Check sheet for the modelled part. Datum: model origin and axes. Units: mm. Face numbers are marked on the shaded views. A direction names the side the tool comes from. Give positions to 0.01 mm unless a question says otherwise; leave off trailing zeros. Order: outer loops, then holes, each group sorted by start corner. A loop starts at its lowest first (then second) coordinate and runs counter-clockwise, first axis right, second up. Notation, with made-up numbers: (-15, -4.5) -> (12, -4.5) arc R35 ccw to (12, 34.5) -> close; hole circle Ø7 at (21.5, 38). An arc over 180 degrees is marked (long way). Answer in a Markdown table with one row per item. Add a question column.
(1) Cross-section at B-B (x = 8.5). Record the cut outline in (y, z).
(2) Release check for a two-part mould opening along X. For the marked faces 1, 2, 3 and 4 record: released by +X, released by -X, zero draft, split by the parting line, or undercut.
(3) Cross-section at D-D (x = 3.5). Record the cut outline in (y, z), then the cut area to 3 significant figures.
(4) Set-up check for the marked faces 5, 6, 7 and 8: record each of +Z, -Z, +X, -X, +Y, -Y from which the full face is reachable in a straight line by a thin tool's end or side.
(5) Cross-section at C-C (z = 5). Record the cut outline in (x, y), then the cut area to 3 significant figures.
(6) Go/stop test with flat-tipped pins: pin 1 (3.5 mm diameter, centred on x = 6, y = -0.5, fed in from +Z); pin 2 (1 mm diameter, centred on x = 8, y = 13.5, fed in from -Z); pin 3 (1 mm diameter, centred on x = 6.5, y = 13.5, fed in from +Z). Record where each tip stops, or that it passes through.
(7) Cross-section at A-A (y = 0). Record the cut outline in (x, z), then the cut area to 3 significant figures.
(8) Thickness scan on L1, parallel to Z at x = 8, y = 0.5; L2, parallel to Z at x = 8.5, y = -3; L3, parallel to Y at x = 8, z = 5. Record the ranges inside material, lowest first. Write a range as [from, to].
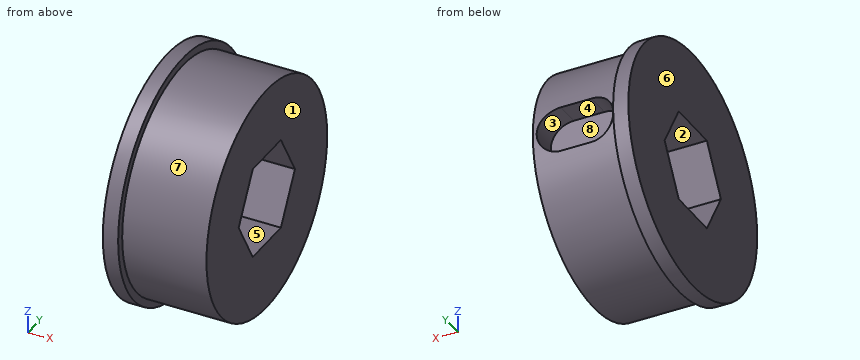
```python
from build123d import *

# Parameters (mm, degrees)
CUT_EXTRUDE1_DEPTH = 27.095976701
CUT_EXTRUDE2_DEPTH = 3.5


with BuildPart() as part:
    # Sketch1 → Revolve1 (revolve)
    with BuildSketch(Plane.XY):
        Polygon((0, 0), (0, 16), (2, 16), (2, 15), (13, 15), (13, 0), align=None)
    revolve(axis=Axis((13, 0, 0), (-1, 0, 0)))

    # Sketch2 → Cut-Extrude1 (cut, through all)
    with BuildSketch(Plane(origin=(13, 0, 0), x_dir=(0, 0, -1), z_dir=(1, 0, 0))):
        Polygon((0, 7), (-6.062177826, 3.5), (-6.062177826, -3.5), (0, -7), (6.062177826, -3.5), (6.062177826, 3.5), align=None)
    extrude(amount=-CUT_EXTRUDE1_DEPTH, mode=Mode.SUBTRACT)

    # Sketch3 → Cut-Extrude2 (cut)
    with BuildSketch(Plane(origin=(0, 15, 0), x_dir=(1, 0, 0), z_dir=(0, 1, 0))):
        with BuildLine():
            Line((5.5, 3), (9.5, 3))
            ThreePointArc((9.5, 3), (12.5, 0), (9.5, -3))
            Line((9.5, -3), (5.5, -3))
            ThreePointArc((5.5, -3), (2.5, 0), (5.5, 3))
        make_face()
    extrude(amount=-CUT_EXTRUDE2_DEPTH, mode=Mode.SUBTRACT)


solid = part.part
```
Answer below:
| question | item | result |
|---|---|---|
| 1 | outline | (11.5, -3) -> (11.5, 3) -> (14.7, 3) arc R15 ccw (long way) to (14.7, -3) -> close; hole (-7, 0) -> (-3.5, -6.06) -> (3.5, -6.06) -> (7, 0) -> (3.5, 6.06) -> (-3.5, 6.06) -> close |
| 2 | face 1 | released by +X |
| 2 | face 2 | zero draft |
| 2 | face 3 | undercut |
| 2 | face 4 | undercut |
| 3 | outline | (11.5, -2.24) -> (11.5, 2.24) -> (14.83, 2.24) arc R15 ccw (long way) to (14.83, -2.24) -> close; hole (-7, 0) -> (-3.5, -6.06) -> (3.5, -6.06) -> (7, 0) -> (3.5, 6.06) -> (-3.5, 6.06) -> close |
| 3 | area | 564 mm² |
| 4 | face 5 | +X, -X |
| 4 | face 6 | +Z, -Z, -X, +Y, -Y |
| 4 | face 7 | +X |
| 4 | face 8 | +Y |
| 5 | outline | (0, -15.2) -> (2, -15.2) -> (2, -14.14) -> (13, -14.14) -> (13, -4.11) -> (0, -4.11) -> close; (0, 4.11) -> (13, 4.11) -> (13, 14.14) -> (2, 14.14) -> (2, 15.2) -> (0, 15.2) -> close |
| 5 | area | 265 mm² |
| 6 | pin 1 | stops at z = 15 |
| 6 | pin 2 | stops at z = -7.48 |
| 6 | pin 3 | stops at z = 7.48 |
| 7 | outline | (0, -16) -> (2, -16) -> (2, -15) -> (13, -15) -> (13, -6.06) -> (0, -6.06) -> close; (0, 6.06) -> (13, 6.06) -> (13, 15) -> (2, 15) -> (2, 16) -> (0, 16) -> close |
| 7 | area | 236 mm² |
| 8 | L1 | z = [-14.99, -6.06], [6.06, 14.99] |
| 8 | L2 | z = [-14.7, -6.06], [6.06, 14.7] |
| 8 | L3 | y = [-14.14, -4.11], [4.11, 14.14] |
